```python
from build123d import *
from OCP.BRepFilletAPI import BRepFilletAPI_MakeChamfer

# Parameters (mm, degrees)
BOSS_EXTRUDE1_DEPTH = 20
CHAMFER1_SIZE       = 20
CHAMFER1_SIZE_2     = 14.004150764
SHELL1_DEPTH        = 15
SHELL1_DRAFT        = 35
CUT_EXTRUDE2_DEPTH  = 129.840987267


# Read off the part's stored shape, not the designer's step: Shell1
with BuildPart() as part:
    # Sketch1 → Boss-Extrude1 (new body)
    with BuildSketch(Plane(origin=(0, 0, 0), x_dir=(1, 0, 0), z_dir=(0, 1, 0))):
        Polygon((90, -37.279220614), (90, 37.279220614), (37.279220614, 90), (-37.279220614, 90), (-90, 37.279220614), (-90, -37.279220614), (-37.279220614, -90), (37.279220614, -90), align=None)
    extrude(amount=BOSS_EXTRUDE1_DEPTH)

    # Chamfer1
    chamfer1_edges_1 = [part.edges().sort_by_distance(p)[0] for p in [
        (0, 20, 90),
    ]]
    chamfer1_side_1 = [part.faces().sort_by_distance(p)[0] for p in [
        (0, 19.719916985, 90),
    ]]
    chamfer1_edges_2 = [part.edges().sort_by_distance(p)[0] for p in [
        (-63.639610307, 20, 63.639610307),
    ]]
    chamfer1_side_2 = [part.faces().sort_by_distance(p)[0] for p in [
        (-63.639610307, 19.719916985, 63.639610307),
    ]]
    chamfer1_edges_3 = [part.edges().sort_by_distance(p)[0] for p in [
        (-90, 20, 0),
    ]]
    chamfer1_side_3 = [part.faces().sort_by_distance(p)[0] for p in [
        (-90, 19.719916985, 0),
    ]]
    chamfer1_edges_4 = [part.edges().sort_by_distance(p)[0] for p in [
        (-63.639610307, 20, -63.639610307),
    ]]
    chamfer1_side_4 = [part.faces().sort_by_distance(p)[0] for p in [
        (-63.639610307, 19.719916985, -63.639610307),
    ]]
    chamfer1_edges_5 = [part.edges().sort_by_distance(p)[0] for p in [
        (0, 20, -90),
    ]]
    chamfer1_side_5 = [part.faces().sort_by_distance(p)[0] for p in [
        (0, 19.719916985, -90),
    ]]
    chamfer1_edges_6 = [part.edges().sort_by_distance(p)[0] for p in [
        (63.639610307, 20, -63.639610307),
    ]]
    chamfer1_side_6 = [part.faces().sort_by_distance(p)[0] for p in [
        (63.639610307, 19.719916985, -63.639610307),
    ]]
    chamfer1_edges_7 = [part.edges().sort_by_distance(p)[0] for p in [
        (90, 20, 0),
    ]]
    chamfer1_side_7 = [part.faces().sort_by_distance(p)[0] for p in [
        (90, 19.719916985, 0),
    ]]
    chamfer1_edges_8 = [part.edges().sort_by_distance(p)[0] for p in [
        (63.639610307, 20, 63.639610307),
    ]]
    chamfer1_side_8 = [part.faces().sort_by_distance(p)[0] for p in [
        (63.639610307, 19.719916985, 63.639610307),
    ]]
    chamfer1 = BRepFilletAPI_MakeChamfer(part.part.solid().wrapped)
    for e in chamfer1_edges_1:
        chamfer1.Add(CHAMFER1_SIZE - 0.0001, CHAMFER1_SIZE_2 - 0.0001, e.wrapped, chamfer1_side_1[0].wrapped)
    for e in chamfer1_edges_2:
        chamfer1.Add(CHAMFER1_SIZE - 0.0001, CHAMFER1_SIZE_2 - 0.0001, e.wrapped, chamfer1_side_2[0].wrapped)
    for e in chamfer1_edges_3:
        chamfer1.Add(CHAMFER1_SIZE - 0.0001, CHAMFER1_SIZE_2 - 0.0001, e.wrapped, chamfer1_side_3[0].wrapped)
    for e in chamfer1_edges_4:
        chamfer1.Add(CHAMFER1_SIZE - 0.0001, CHAMFER1_SIZE_2 - 0.0001, e.wrapped, chamfer1_side_4[0].wrapped)
    for e in chamfer1_edges_5:
        chamfer1.Add(CHAMFER1_SIZE - 0.0001, CHAMFER1_SIZE_2 - 0.0001, e.wrapped, chamfer1_side_5[0].wrapped)
    for e in chamfer1_edges_6:
        chamfer1.Add(CHAMFER1_SIZE - 0.0001, CHAMFER1_SIZE_2 - 0.0001, e.wrapped, chamfer1_side_6[0].wrapped)
    for e in chamfer1_edges_7:
        chamfer1.Add(CHAMFER1_SIZE - 0.0001, CHAMFER1_SIZE_2 - 0.0001, e.wrapped, chamfer1_side_7[0].wrapped)
    for e in chamfer1_edges_8:
        chamfer1.Add(CHAMFER1_SIZE - 0.0001, CHAMFER1_SIZE_2 - 0.0001, e.wrapped, chamfer1_side_8[0].wrapped)
    add(Compound.cast(chamfer1.Shape()), mode=Mode.REPLACE)  # a hair under: the kernel refuses the full size


with BuildPart() as shell1_tool:
    # Shell1 outline → Shell1 (with draft: the straight prism first)
    with BuildSketch(Plane(origin=(0, 15, 0), x_dir=(1, 0, 0), z_dir=(0, 1, 0))):
        Polygon((-30.400381775, -73.393013983), (30.400381775, -73.393013983), (73.393013983, -30.400381775), (73.393013983, 30.400381775), (30.400381775, 73.393013983), (-30.400381775, 73.393013983), (-73.393013983, 30.400381775), (-73.393013983, -30.400381775), align=None)
    extrude(amount=-SHELL1_DEPTH)
    # Shell1: the draft: its side faces are tilted about the plane it starts from
    shell1_sides = [shell1_tool.faces().sort_by_distance(p)[0] for p in [
        (0, 7.5, 73.393013983),
        (51.896697879, 7.5, 51.896697879),
        (73.393013983, 7.5, 0),
        (51.896697879, 7.5, -51.896697879),
        (0, 7.5, -73.393013983),
        (-51.896697879, 7.5, -51.896697879),
        (-73.393013983, 7.5, 0),
        (-51.896697879, 7.5, 51.896697879),
    ]]
    draft(shell1_sides, Plane(origin=(0, 15, 0), x_dir=(1, 0, 0), z_dir=(0, 1, 0)), SHELL1_DRAFT)


with BuildPart() as part_1:
    add(part.part)

    # Shell1: cut by shell1_tool
    add(shell1_tool.part, mode=Mode.SUBTRACT)

    # Sketch2 → Cut-Extrude2 (cut, through all)
    with BuildSketch(Plane(origin=(0, 20, 0), x_dir=(1, 0, 0), z_dir=(0, 1, 0))):
        Polygon((20.710678119, 50), (-20.710678119, 50), (-50, 20.710678119), (-50, -20.710678119), (-20.710678119, -50), (20.710678119, -50), (50, -20.710678119), (50, 20.710678119), align=None)
    extrude(amount=-CUT_EXTRUDE2_DEPTH, mode=Mode.SUBTRACT)


solid = part_1.part
```
CAD build for the part. Positions are in the model's coordinates, mm. A direction names the side the tool comes from. Coordinates: 2 decimals unless noted, no trailing zeros. Order: outer loops, then holes, each group sorted by start corner. A loop starts at its lowest first (then second) coordinate and runs counter-clockwise, first axis right, second up. Notation, with made-up numbers: (-10, 31.5) - (13, 31.5) arc R36 cw to (13, 68.5) - close; hole circle Ø2 at (35.5, 66.5). An arc over 180 degrees is marked (long way). Answer in a Markdown table with one row per item.
1. 3-axis set-ups, long thin cutter, end or side, ignore diameter. For faces 1 (the face through (35.15, 17.54, 35.56)), 2 (the face through (-0.487, 7.605, 78.571)), 3 (the face through (60, 0, 60)): which of +Z, -Z, +X, -X, +Y, -Y reach the whole face in a straight line?
Answer:
| item | result |
|---|---|
| face 1 | +Y, -Y |
| face 2 | -Y |
| face 3 | +Z, -Z, +X, -X, -Y |
2. Pull direction X, two halves, no side cores. Call faces 4 (the face through (58.99, 10.14, -58.25)), 5 (the face through (-1, 20, -52)), 6 (the face through (-35.56, 17.54, 35.15)): +X half, -X half, draft (parallel to the pull), parting line (faces both ways), or undercut.
Answer:
| item | result |
|---|---|
| face 4 | +X half |
| face 5 | draft |
| face 6 | undercut |
3. Slice it at C-C, the plane y = 17.25. List the corners of the cut face in (x, z), then the cut area to 3 significant figures.
Answer:
| item | result |
|---|---|
| outline | (-77.92, -32.28) - (-32.28, -77.92) - (32.28, -77.92) - (77.92, -32.28) - (77.92, 32.28) - (32.28, 77.92) - (-32.28, 77.92) - (-77.92, 32.28) - close; hole (-50, -20.71) - (-20.71, -50) - (20.71, -50) - (50, -20.71) - (50, 20.71) - (20.71, 50) - (-20.71, 50) - (-50, 20.71) - close |
| area | 11,800 mm² |
4. Flat gauge pins, fed straight in: P1, Ø6, axis at x = -69.5, z = -19.5, coming from the -Y side; P2, Ø3, axis at x = 47, z = 4.5, coming from the -Y side; P3, Ø6, axis at x = -14, y = 14, coming from the -Z side; P4, Ø1.5, axis at x = 7, y = 17, coming from the -Z side. Where does each tip first touch, or does it go through?
Answer:
| item | result |
|---|---|
| P1 | y = 15 |
| P2 | through |
| P3 | z = -82.3 |
| P4 | z = -78.62 |
5. Drill centre lines: L1, parallel to Y at x = -54, z = 12; L2, parallel to Z at x = 19, y = 14.5; L3, parallel to X at y = 16.5, z = -13. Where is each one in solid material? Low to high. Write a range as from..to.
Answer:
| item | result |
|---|---|
| L1 | 15..20 |
| L2 | -79.85..-73.74, 73.74..79.85 |
| L3 | -78.45..-50, 50..78.45 |
